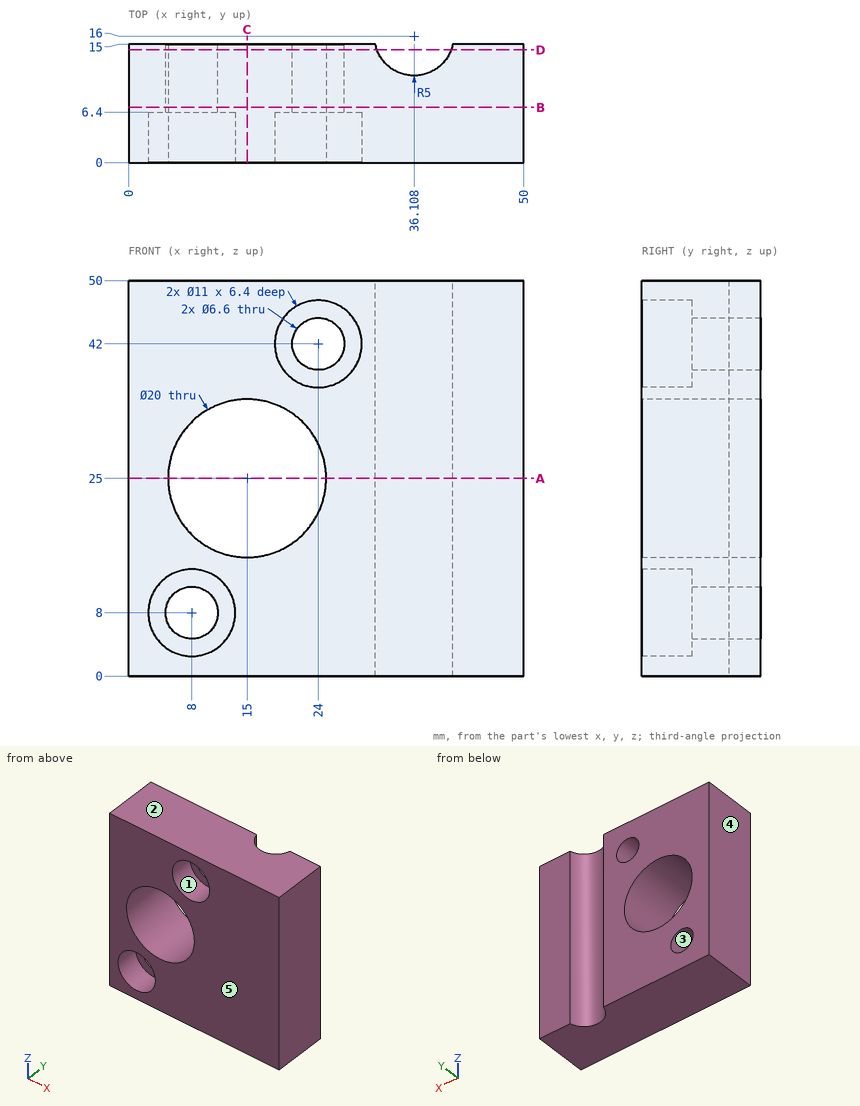
Drawing for the job (mm, zero at the part's lowest x, y, z). A direction names the side the tool comes from. Round coordinates to 2 decimals unless told otherwise and drop trailing zeros. Write each loop counter-clockwise with the first axis right and the second up, starting at its lowest first coordinate (ties: lowest second). Pieces come first, ordered by that corner, then holes.
Item 1: Band-saw the part on D-D on y = 14.25. Write the cut outline in (x, z) (1 decimal), then the cut area to 3 significant figures.
Filled in:
outline: (0, 0) - (31.4, 0) - (31.4, 50) - (0, 50) - close; (40.8, 0) - (50, 0) - (50, 50) - (40.8, 50) - close; hole circle Ø6.6 at (8, 8); hole circle Ø20 at (15, 25); hole circle Ø6.6 at (24, 42)
area: 1,650 mm2
Item 2: Drill centre lines: L1, parallel to X at y = 3.25, z = 42; L2, parallel to X at y = 12.25, z = 8.5 (1 decimal); L3, parallel to X at y = 10, z = 42. Where is each one in solid material? Low to high.
Filled in:
L1: x = 0 to 18.5, 29.5 to 50
L2: x = 0 to 4.7, 11.3 to 32.8, 39.4 to 50
L3: x = 0 to 20.7, 27.3 to 50
Item 3: Band-saw the part on A-A on z = 25. Write the cut outline in (x, y).
Filled in:
outline: (0, 0) - (5, 0) - (5, 15) - (0, 15) - close; (25, 0) - (50, 0) - (50, 15) - (41.01, 15) arc R5 cw to (31.21, 15) - (25, 15) - close
Item 4: Band-saw the part on B-B on y = 7. Write the cut outline in (x, z), then the cut area to 3 significant figures.
Filled in:
outline: (0, 0) - (50, 0) - (50, 50) - (0, 50) - close; hole circle Ø6.6 at (8, 8); hole circle Ø20 at (15, 25); hole circle Ø6.6 at (24, 42)
area: 2,120 mm2
Item 5: Mould opens along X. For the marked faces 3, 4 and 5 say: released by +X, released by -X, zero draft, split by the parting line, or undercut.
Filled in:
face 3: undercut
face 4: released by -X
face 5: zero draft
Item 6: Tool access for the marked faces 1 and 2: list every direction of +Z, -Z, +X, -X, +Y, -Y with a clear straight run to the whole face (end or side of a thin tool).
Filled in:
face 1: -Y
face 2: +Z, +X, -X, +Y, -Y
Item 7: Band-saw the part on C-C on x = 15. Write the cut outline in (y, z).
Filled in:
outline: (0, 0) - (15, 0) - (15, 15) - (0, 15) - close; (0, 35) - (15, 35) - (15, 50) - (0, 50) - close
